from build123d import *

# Parameters (mm, degrees)
SKETCH_1_R      = 4
EXTRUDE_1_DEPTH = 150
SKETCH_2_W      = 12
SKETCH_2_H      = 4
EXTRUDE_2_DEPTH = 10


with BuildPart() as part:
    # Эскиз1 → Бобышка-Вытянуть1 (new body)
    with BuildSketch(Plane.XY):
        Circle(SKETCH_1_R)
    extrude(amount=EXTRUDE_1_DEPTH)

    # Эскиз2 → Бобышка-Вытянуть2 (add)
    with BuildSketch(Plane(origin=(0, 0, 0), x_dir=(-1, 0, 0), z_dir=(0, 0, -1))):
        Rectangle(SKETCH_2_W, SKETCH_2_H)
    extrude(amount=-EXTRUDE_2_DEPTH)


solid = part.part
Read the model definition and answer for the solid it produces. Units are mm, in the model's axes. A direction names the side the tool comes from. Round coordinates to 2 decimals unless told otherwise and drop trailing zeros. Write each loop counter-clockwise with the first axis right and the second up, starting at its lowest first coordinate (ties: lowest second). Pieces come first, ordered by that corner, then holes. Notation, with made-up numbers: (-18, 82.5) - (41, 82.5) arc R23 cw to (41, 96.5) - close; hole circle Ø9 at (46.5, -23). An arc over 180 degrees is marked (long way). Use a Markdown table: item, result.
(1) Each of these flat-tipped pins is pushed along its axis until it touches: pin 1 Ø3 at (y, z) = (-2, 86) entering from -X; pin 2 Ø2 at (y, z) = (1, 69.5) entering from +X; pin 3 Ø2 at (x, z) = (4.5, 6.5) entering from +Y. Where does it stop, or does it pass through?
Reported:
| item | result |
|---|---|
| pin 1 | x = -3.97 |
| pin 2 | x = 4 |
| pin 3 | y = 2 |
(2) Straight lines are drawn through the part: line 1 along X through (y, z) = (2, 37); line 2 along Z through (x, y) = (-5.5, -1.25); line 3 along X through (y, z) = (3.25, 26). For each, find the intervals that lie inside material, in ascending order. Write a range as [from, to].
Reported:
| item | result |
|---|---|
| line 1 | [-3.46, 3.46] |
| line 2 | [0, 10] |
| line 3 | [-2.33, 2.33] |
(3) The part is cut by section B-B (z = 66). Write down the section's boundary in (x, y).
Reported:
| item | result |
|---|---|
| outline | circle Ø8 at (0, 0) |
(4) The part is cut by section A-A (y = 0). Write down the section's boundary in (x, z), then the cut area to 3 significant figures.
Reported:
| item | result |
|---|---|
| outline | (-6, 0) - (6, 0) - (6, 10) - (4, 10) - (4, 150) - (-4, 150) - (-4, 10) - (-6, 10) - close |
| area | 1,240 mm2 |
(5) Which of the six approach directions +Z, -Z, +X, -X, +Y, -Y give full straight-line access (tool end or side, diameter ignored) to faces 1 (the flat face through (-5, -2, 5)), 2 (the flat face through (-5, 2, 5)), 3 (the cylindrical face through (-4, 0, 74))?
Reported:
| item | result |
|---|---|
| face 1 | +Z, -Z, -X, -Y |
| face 2 | +Z, -Z, -X, +Y |
| face 3 | +Z |
(6) The part is cut by section C-C (x = 2). Write down the section's boundary in (y, z), then the cut area to 3 significant figures.
Reported:
| item | result |
|---|---|
| outline | (-3.46, 0) - (3.46, 0) - (3.46, 150) - (-3.46, 150) - close |
| area | 1,040 mm2 |
